Read the model definition and answer for the solid it produces. Units are mm, in the model's axes. Face numbers are marked on the shaded views. A direction names the side the tool comes from. Give positions to 0.01 mm unless a question says otherwise; leave off trailing zeros. Loops run counter-clockwise (first coordinate to the right, second up) from the corner with the lowest first, then second, coordinate; pieces in that order, holes last. Notation, with made-up numbers: (65.25, 86) - (83.25, 86) arc R22 ccw to (83.25, 109) - close; hole circle Ø11 at (3.25, 3). An arc over 180 degrees is marked (long way). Use a Markdown table: item, result. Add a question column.
Item 1: A cutting plane is placed at D-D (x = 0). Determine the outline of the cut face in (y, z), plus the area to 3 significant figures.
Item 2: A cutting plane is placed at B-B (z = -5). Determine the outline of the cut face in (x, y).
Item 3: Each of these flat-tipped pins is pushed along its axis until it touches: P1, Ø10, axis at x = -18.5, y = 22.5, coming from the -Z side; P2, Ø10, axis at y = 37, z = -7, coming from the -X side; P3, Ø1.5, axis at y = 29, z = 9, coming from the +X side; P4, Ø10, axis at y = 14, z = 1, coming from the -X side. Where does it stop, or does it pass through?
Item 4: Which of the six approach directions +Z, -Z, +X, -X, +Y, -Y give full straight-line access (tool end or side, diameter ignored) to the marked faces 1 and 2?
Item 5: Consider probe 1 along Y at (x, z) = (-32, -10.35); probe 2 along Y at (x, z) = (0, 10.5); probe 3 along Y at (x, z) = (-21.5, 9). Determine where each line is inside the solid, lowest interval first. Write a range as [from, to].
Item 6: For a pull along X with two mould halves and no side action, classify the marked faces 3, 4, 5 and 6 as +X half, -X half, draft (parallel to the pull), parting line (faces both ways), or undercut.
Item 7: A cutting plane is placed at C-C (y = 7). Give the number of separate pieces and of enclosed holes in the cut face, plus the area to 3 significant figures.
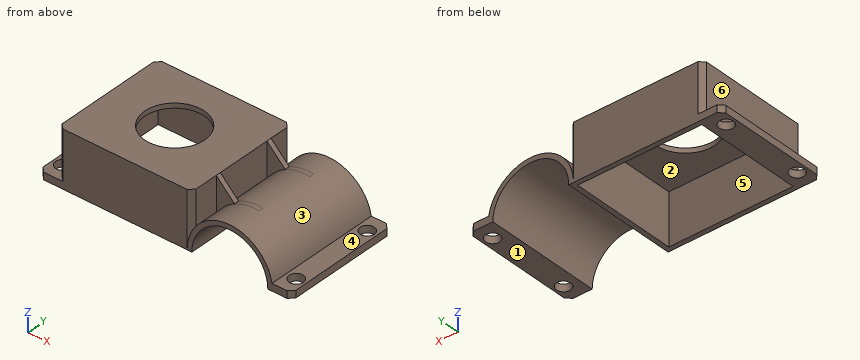
Autodesk Inventor part; units mm, degrees
ref_plane "YZ Plane" through (0, 0, 0) normal (1, 0, 0) x (0, 1, 0)
ref_plane "XZ Plane" through (0, 0, 0) normal (0, 1, 0) x (-1, 0, 0)
ref_plane "XY Plane" through (0, 0, 0) normal (0, 0, 1) x (1, 0, 0)
sketch "Esboço1" plane through (0, 0, 0) normal (0, 1, 0) x (-1, 0, 0)
  line L0 (-28, -11.75) -> (28, -11.75)
  line L1 (28, -11.75) -> (28, 11.75)
  line L2 (28, 11.75) -> (-28, 11.75)
  line L3 (-28, 11.75) -> (-28, -11.75)
  line L4 (-28, -11.75) -> (28, 11.75) construction
  line L5 (28, -11.75) -> (-28, 11.75) construction
  point P0 (0, 0)
  dimension "d0" = 56
  dimension "d1" = 23.5
extrude "Extrusão1" add sketch "Esboço1" along normal blind 49
sketch "Esboço2" plane through (28, 0, -11.75) normal (0, 0, -1) x (-1, 0, 0)
  line L0 (0, 49) -> (56, 49)
  line L1 (0, 49) -> (-33.75, 49)
  line L2 (-33.75, 49) -> (-33.75, 0)
  line L3 (0, 0) -> (56, 0)
  line L4 (-33.75, 0) -> (0, 0)
  line L5 (0, 0) -> (0, 49)
  point P0 (28, 0)
  dimension "d4" = 33.75
extrude "Extrusão2" add sketch "Esboço2" against normal blind 17.875
sketch "Esboço3" plane through (0, 49, 0) normal (0, 1, 0) x (1, 0, 0)
  line L0 (-28, 11.75) -> (61.75, 11.75)
  line L1 (61.75, 11.75) -> (59.75, 11.75)
  line L2 (59.75, 11.75) -> (43.875, 11.75)
  circle A0 centre (43.875, 11.75) radius 15.875
  point P0 (0, 0)
  dimension "d7" = 2
  dimension "d8" = 15.875
extrude "Extrusão3" cut sketch "Esboço3" against normal blind 49
sketch "Esboço4" plane through (61.75, 0, -11.75) normal (0, 0, -1) x (-1, 0, 0)
  line L0 (0, 49) -> (33.75, 49)
  line L1 (33.75, 0) -> (0, 0)
  line L2 (0, 49) -> (0, 0)
  line L3 (0, 0) -> (-8, 0)
  line L4 (-8, 0) -> (-8, 49)
  line L5 (-8, 49) -> (0, 49)
  line L6 (-4, 0) -> (-4, 7)
  line L7 (-4, 49) -> (-4, 42)
  circle A0 centre (-4, 42) radius 3
  circle A1 centre (-4, 7) radius 3
  point P0 (61.75, 0)
  dimension "d11" = 8
  dimension "d12" = 7
  dimension "d13" = 7
  dimension "d14" = 6
  dimension "d15" = 6
extrude "Extrusão4" add sketch "Esboço4" against normal blind 3
sketch "Esboço5" plane through (0, 49, 0) normal (0, 1, 0) x (1, 0, 0)
  arc A0 (28, 11.75) -> (59.75, 11.75) centre (43.875, 11.75) ccw
  circle A1 centre (43.875, 11.75) radius 17.875
  line L0 (61.75, -6.125) -> (28, -6.125)
  line L1 (69.75, 8.75) -> (61.75, 8.75)
  line L2 (61.75, 8.75) -> (61.4965, 8.75)
  line L3 (61.75, 8.75) -> (61.75, -6.125)
  line L4 (43.875, -6.125) -> (61.75, -6.125)
  line L5 (28, -11.75) -> (28, -6.125)
  line L6 (43.875, -6.125) -> (28, -6.125)
  line L7 (28, -6.125) -> (28, 3.5342)
  point P0 (0, 0)
extrude "Extrusão5" cut sketch "Esboço5" against normal blind 49 contours A1 L0 L7 | L2 L3 L0 A1
sketch "Esboço6" plane through (-28, 0, -11.75) normal (0, 0, -1) x (-1, 0, 0)
  line L0 (0, 0) -> (0, 49)
  line L1 (0, 49) -> (0, 0)
  line L2 (0, 0) -> (8, 0)
  line L3 (8, 0) -> (8, 49)
  line L4 (8, 49) -> (0, 49)
  line L5 (4, 49) -> (4, 42)
  line L6 (4, 0) -> (4, 7)
  circle A0 centre (4, 7) radius 3
  circle A1 centre (4, 42) radius 3
  point P0 (-28, 0)
  dimension "d20" = 8
  dimension "d21" = 7
  dimension "d22" = 7
  dimension "d23" = 6
  dimension "d24" = 6
extrude "Extrusão6" add sketch "Esboço6" against normal blind 3
sketch "Esboço8" plane through (28, 0, -11.75) normal (0, 0, -1) x (-1, 0, 0)
  line L0 (0, 49) -> (0, 0)
  line L1 (0, 49) -> (0, 47)
  line L2 (0, 47) -> (2, 47)
  line L3 (2, 47) -> (2, 2)
  line L4 (2, 47) -> (47, 47) construction
  line L5 (2, 2) -> (54, 2)
  line L6 (2, 2) -> (54, 2) construction
  line L7 (54, 2) -> (54, 47)
  line L8 (54, 47) -> (2, 47)
  point P0 (28, 0)
  dimension "d27" = 2
  dimension "d28" = 2
  dimension "d29" = 45
  dimension "d30" = 90
  dimension "d31" = 52
  dimension "d32" = 0
extrude "Extrusão7" cut sketch "Esboço8" against normal blind 21.5
sketch "Esboço9" plane through (-28, 0, 11.75) normal (0, 0, 1) x (1, 0, 0)
  circle A0 centre (28, 24.5) radius 12.5
  point P0 (28, 0)
  dimension "d35" = 25
extrude "Extrusão8" cut sketch "Esboço9" against normal blind 2
sketch "Esboço10" plane through (28, 0, 11.75) normal (1, 0, 0) x (0, 0, -1)
  line L0 (0, 0) -> (0, 49)
  line L1 (0, 49) -> (0, 37)
  line L2 (0, 0) -> (0, 12)
  line L3 (0, 12) -> (16, 12)
  line L4 (16, 12) -> (16, 14)
  line L5 (16, 14) -> (0, 14)
  line L6 (0, 12) -> (0, 14)
  line L7 (0, 37) -> (16, 37)
  line L8 (16, 37) -> (16, 39)
  line L9 (16, 39) -> (0, 39)
  point P0 (11.75, 0)
  dimension "d38" = 12
  dimension "d41" = 12
  dimension "d42" = 16
  dimension "d43" = 2
  dimension "d44" = 16
  dimension "d45" = 2
extrude "Extrusão9" add sketch "Esboço10" along normal blind 17.875
sketch "Esboço11" plane through (28, 39, 11.75) normal (0, 1, 0) x (1, 0, 0)
  arc A0 (0, 15.2842) -> (33.4965, 20.5) centre (15.875, 23.5) ccw
  arc A1 (0, 23.5) -> (31.75, 23.5) centre (15.875, 23.5) ccw
  line L0 (17.875, 0) -> (17.875, 5.7372)
  line L1 (17.875, 5.7372) -> (17.875, 0)
  line L2 (0, 0) -> (17.875, 0)
  line L3 (17.875, 0) -> (0, 0)
  line L4 (0, 0) -> (7.6367, 7.6367)
  arc A2 (0, 15.2842) -> (17.875, 5.7372) centre (15.875, 23.5) ccw
  arc A3 (7.6367, 7.6367) -> (17.875, 5.7372) centre (15.875, 23.5) ccw
  line L5 (1.8834, 16) -> (17.875, 16)
  line L6 (1.8834, 16) -> (17.875, 16)
  line L7 (17.875, 16) -> (17.875, 7.7515)
  line L8 (17.875, 16) -> (17.875, 7.7515)
  arc A4 (1.8834, 16) -> (17.875, 7.7515) centre (15.875, 23.5) ccw
  point P0 (-28, 11.75)
  dimension "d48" = 45
extrude "Extrusão10" cut sketch "Esboço11" against normal blind 27.875
chamfer "Chanfro1" distance 2 angle 45 8 edges at (28, 49, 4.1079) (28, 0, 4.1079) (-28, 0, 1.5) (-28, 49, 1.5) (69.75, 49, -10.25) (69.75, 0, -10.25) (-36, 49, -10.25) (-36, 0, -10.25)
properties part number "KS  Dianteiro Front"
Geometry says:
| question | item | result |
|---|---|---|
| 1 | outline | (0, -11.75) - (2, -11.75) - (2, 9.75) - (12, 9.75) - (12, 11.75) - (0, 11.75) - close; (37, 9.75) - (47, 9.75) - (47, -11.75) - (49, -11.75) - (49, 11.75) - (37, 11.75) - close |
| 1 | area | 134 mm² |
| 2 | outline | (-28, 2) - (-26, 0) - (26, 0) - (27.32, 1.32) - (27.32, 0) - (29.51, 0) - (29.51, 49) - (27.32, 49) - (27.32, 47.68) - (26, 49) - (-26, 49) - (-28, 47) - close; (58.24, 0) - (60.43, 0) - (60.43, 49) - (58.24, 49) - close; hole (-26, 2) - (26, 2) - (26, 47) - (-26, 47) - close |
| 3 | P1 | z = 9.75 |
| 3 | P2 | x = -36 |
| 3 | P3 | x = 28 |
| 3 | P4 | x = -28 |
| 4 | face 1 | -Z, +X, -X, +Y, -Y |
| 4 | face 2 | -Z |
| 5 | probe 1 | [0, 4], [10, 39], [45, 49] |
| 5 | probe 2 | [0, 12], [37, 49] |
| 5 | probe 3 | [0, 2], [47, 49] |
| 6 | face 3 | undercut |
| 6 | face 4 | draft |
| 6 | face 5 | undercut |
| 6 | face 6 | -X half |
| 7 | separate pieces | 3 |
| 7 | enclosed holes | 0 |
| 7 | area | 305 mm² |
